from build123d import *

# Parameters (mm, degrees)
ESQUISSE1_W             = 20
ESQUISSE1_H             = 10
BOSS_EXTRU_1_DEPTH      = 5.842
ESQUISSE2_W             = 0.635
ESQUISSE2_H             = 3.175
ESQUISSE2_W_2           = 0.70971707
BOSS_EXTRU_3_DEPTH      = 1.5875
ESQUISSE3_R             = 1
ENL_V_MAT_EXTRU_1_DEPTH = 15.176021621


with BuildPart() as part:
    # Esquisse1 → Boss.-Extru.1 (new body)
    with BuildSketch(Plane(origin=(0, 0, 0), x_dir=(1, 0, 0), z_dir=(0, 1, 0))):
        Rectangle(ESQUISSE1_W, ESQUISSE1_H)
    extrude(amount=BOSS_EXTRU_1_DEPTH)

    # Esquisse2 → Boss.-Extru.3 (add, symmetric)
    with BuildSketch(Plane(origin=(0, 2.921, 0), x_dir=(-1, 0, 0), z_dir=(0, -1, 0))):
        with Locations((8.4125, -6.5875)):
            Rectangle(ESQUISSE2_W, ESQUISSE2_H)
        with Locations((-8.4125, -6.5875)):
            Rectangle(ESQUISSE2_W, ESQUISSE2_H)
        with Locations((0, -6.5875)):
            Rectangle(ESQUISSE2_W_2, ESQUISSE2_H)
    extrude(amount=BOSS_EXTRU_3_DEPTH, both=True)

    # Esquisse3 → Enlèv. mat.-Extru.1 (cut, through all)
    with BuildSketch(Plane.XZ):
        with Locations(Location((3.5, 2.5, 0), (0, 0, 270))):
            Circle(ESQUISSE3_R)
        with Locations(Location((-3.5, 2.5, 0), (0, 0, 90))):
            Circle(ESQUISSE3_R)
    extrude(amount=-ENL_V_MAT_EXTRU_1_DEPTH, mode=Mode.SUBTRACT)


solid = part.part
Work out the finished part from the listing and answer in its coordinate system (mm). A direction names the side the tool comes from. Give positions to 0.01 mm unless a question says otherwise; leave off trailing zeros. Loops run counter-clockwise (first coordinate to the right, second up) from the corner with the lowest first, then second, coordinate; pieces in that order, holes last. Notation, with made-up numbers: (31, -15.75) -> (85, -15.75) arc R14 ccw to (85, -2.75) -> close; hole circle Ø7 at (10.25, 83). An arc over 180 degrees is marked (long way). Use a Markdown table: item, result. Add a question column.
1. For faces 1 (the flat face through (8.73, 3, 7)), 2 (the flat face through (-8.73, 3, 7)), 3 (the flat face through (-8.095, 3, 7)), determine the directions among +Z, -Z, +X, -X, +Y, -Y from which every point of the face is accessible in a straight line to the end or side of a thin tool.
2. Determine the mould class of faces 4 (the cylindrical face through (-4.176, 2.88, 1.763)), 5 (the flat face through (0.355, 3, 7)), 6 (the flat face through (0, 3, -5)) for opening direction Z: released by +Z, released by -Z, zero draft, split by the parting line, or undercut.
3. Section B-B on z = 2.5 is taken. Determine the outline of the cut face in (x, y).
4. Section C-C on y = 3.9 is taken. Determine the outline of the cut face in (x, z) (3 decimals).
5. Flat-ended cylindrical pins translate along their axes: pin 1 Ø1.6 at (y, z) = (3.5, 6) entering from +X; pin 2 Ø1.2 at (x, z) = (-3.5, 2.5) entering from -Y; pin 3 Ø1 at (y, z) = (3, 6.5) entering from -X; pin 4 Ø0.7 at (x, z) = (-8.5, 7.5) entering from -Y. Find the tip coordinate at first contact, or state that the pin passes through.
6. Section A-A on x = 3.5 is taken. Determine the outline of the cut face in (y, z).
7. Section D-D on x = 0 is taken. Determine the outline of the cut face in (y, z) (1 decimal).
8. Find the intervals of material crossed by probe 1 along X at (y, z) = (2.35, 2.5); probe 2 along X at (y, z) = (4.05, 6.75) (3 decimals); probe 3 along Z at (x, y) = (7.25, 5.25), in increasing order.
Results below:
| question | item | result |
|---|---|---|
| 1 | face 1 | +Z, +X, +Y, -Y |
| 1 | face 2 | +Z, -X, +Y, -Y |
| 1 | face 3 | +Z, +Y, -Y |
| 2 | face 4 | undercut |
| 2 | face 5 | zero draft |
| 2 | face 6 | released by -Z |
| 3 | outline | (-10, 0) -> (-4.5, 0) -> (-4.5, 5.84) -> (-10, 5.84) -> close; (-2.5, 0) -> (2.5, 0) -> (2.5, 5.84) -> (-2.5, 5.84) -> close; (4.5, 0) -> (10, 0) -> (10, 5.84) -> (4.5, 5.84) -> close |
| 4 | outline | (-10, -5) -> (10, -5) -> (10, 5) -> (8.73, 5) -> (8.73, 8.175) -> (8.095, 8.175) -> (8.095, 5) -> (0.355, 5) -> (0.355, 8.175) -> (-0.355, 8.175) -> (-0.355, 5) -> (-8.095, 5) -> (-8.095, 8.175) -> (-8.73, 8.175) -> (-8.73, 5) -> (-10, 5) -> close; hole circle Ø2 at (-3.5, 2.5); hole circle Ø2 at (3.5, 2.5) |
| 5 | pin 1 | stops at x = 8.73 |
| 5 | pin 2 | passes through |
| 5 | pin 3 | stops at x = -8.73 |
| 5 | pin 4 | stops at y = 1.33 |
| 6 | outline | (0, -5) -> (5.84, -5) -> (5.84, 1.5) -> (0, 1.5) -> close; (0, 3.5) -> (5.84, 3.5) -> (5.84, 5) -> (0, 5) -> close |
| 7 | outline | (0, -5) -> (5.8, -5) -> (5.8, 5) -> (4.5, 5) -> (4.5, 8.2) -> (1.3, 8.2) -> (1.3, 5) -> (0, 5) -> close |
| 8 | probe 1 | x = -10 to -4.5, -2.5 to 2.5, 4.5 to 10 |
| 8 | probe 2 | x = -8.73 to -8.095, -0.355 to 0.355, 8.095 to 8.73 |
| 8 | probe 3 | z = -5 to 5 |
